```python
from build123d import *

# Parameters (mm, degrees)
CROQUIS1_W                   = 30
CROQUIS1_H                   = 33.6
SALIENTE_EXTRUIR1_DEPTH      = 3
SALIENTE_EXTRUIR2_DEPTH      = 20
SALIENTE_EXTRUIR2_DEPTH_BACK = 65
CROQUIS2_R                   = 2.5


with BuildPart() as part:
    # Croquis1 → Saliente-Extruir1 (new body)
    with BuildSketch(Plane(origin=(0, 0, 0), x_dir=(0, 0, -1), z_dir=(1, 0, 0))):
        Rectangle(CROQUIS1_W, CROQUIS1_H)
    extrude(amount=SALIENTE_EXTRUIR1_DEPTH)

    # Croquis2 → Saliente-Extruir2 (add, two sides: drawn at the far end of the back side and taken through both)
    with BuildSketch(Plane(origin=(0, 16.8, 0), x_dir=(1, 0, 0), z_dir=(0, 1, 0)).offset(-SALIENTE_EXTRUIR2_DEPTH_BACK)):
        with Locations(Location((1.5, -15, 0), (0, 0, 270))):
            Circle(CROQUIS2_R)
    extrude(amount=SALIENTE_EXTRUIR2_DEPTH + SALIENTE_EXTRUIR2_DEPTH_BACK)


solid = part.part
```
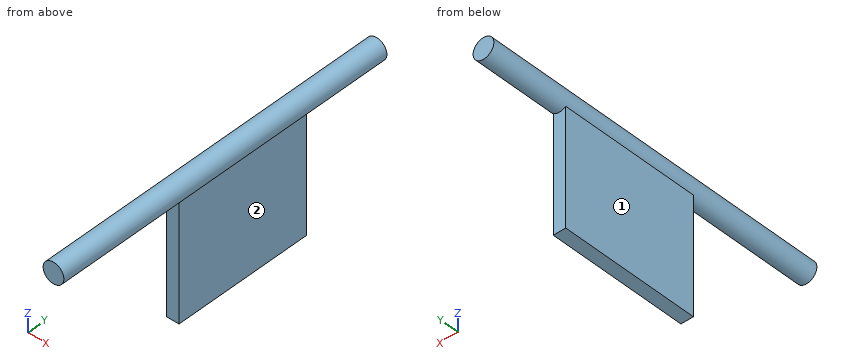
Design review of the part built by this model. Coordinates are the model's own, in mm. Face numbers are marked on the shaded views. A direction names the side the tool comes from. Round coordinates to 2 decimals unless told otherwise and drop trailing zeros. Write each loop counter-clockwise with the first axis right and the second up, starting at its lowest first coordinate (ties: lowest second). Pieces come first, ordered by that corner, then holes. Notation, with made-up numbers: (75.25, 15) -> (84.25, 15) arc R25 ccw to (84.25, 33) -> close; hole circle Ø6 at (22, 18). An arc over 180 degrees is marked (long way). Write item = value, one per line. Start each with the question number.
1) Take a section at A-A, the plane x = 1.5. State the section outline as (y, z) points.
2) Take a section at C-C, the plane z = -7. State the section outline as (x, y) points, plus the area to 3 significant figures.
3) Take a section at B-B, the plane y = 13. State the section outline as (x, z) points, plus the area to 3 significant figures.
4) Tool access review of the marked faces 1 and 2: name each direction out of +Z, -Z, +X, -X, +Y, -Y from which nothing blocks a thin tool from reaching the whole face with its end or side.
5) Clearance check with flat-ended pins moving along their axes: pin 1 (14 mm diameter, centred on y = -4, z = 4, fed in from -X); pin 2 (0.9 mm diameter, centred on x = 1, z = 1, fed in from -Y); pin 3 (10 mm diameter, centred on y = 13, z = -1, fed in from +X). State where each tip first meets the part, or that it passes through.
6) Wall thickness on probe 1 along Y at (x, z) = (0.85, -7.5); probe 2 along Z at (x, y) = (1.7, -7); probe 3 along X at (y, z) = (-14, -11): over which ranges is each line inside the solid? List them lowest first. Write a range as from..to.
7) Take a section at D-D, the plane y = -32.5. State the section outline as (x, z) points.
Results list:
q1.outline = (-48.2, 12.5) -> (-16.8, 12.5) -> (-16.8, -15) -> (16.8, -15) -> (16.8, 12.5) -> (36.8, 12.5) -> (36.8, 17.5) -> (-48.2, 17.5) -> close
q2.outline = (0, -16.8) -> (3, -16.8) -> (3, 16.8) -> (0, 16.8) -> close
q2.area = 101 mm²
q3.outline = (0, -15) -> (3, -15) -> (3, 13) arc R2.5 ccw (long way) to (0, 13) -> close
q3.area = 103 mm²
q4.face_1 = -Z, -X, +Y, -Y
q4.face_2 = -Z, +X, +Y, -Y
q5.pin_1 = 0
q5.pin_2 = -16.8
q5.pin_3 = 3
q6.probe_1 = -16.8..16.8
q6.probe_2 = -15..17.49
q6.probe_3 = 0..3
q7.outline = circle Ø5 at (1.5, 15)
